from build123d import *

# Parameters (mm, degrees)
SWEEP1_PROFILE_R     = 13.49375
CUT_SWEEP1_PROFILE_R = 9.525


with BuildPart() as part:
    # Sweep1: sweep along a curve in space
    with BuildLine() as sweep1_path:
        Line((27.501516454, -11.100021656, -13.942942833), (23.095618699, 7.173839424, -10.851573197))
        add(Edge.make_bspline(
            [(23.095618699, 7.173839424, -10.851573197), (13.261070206, 47.963522462, -3.951225916), (-24.99522441, 69.205871428, 24.49264735), (-71.502710672, 110.316771936, -5.131837889)],
            knots=[0, 0, 0, 0, 1, 1, 1, 1], degree=3))
        Line((-71.502710672, 110.316771936, -5.131837889), (-88.677665299, 125.498797619, -16.07199464))
    # Sweep1 profile (on start of the path) → Sweep1 (sweep)
    with BuildSketch(Plane(origin=(27.501516454, -11.100021656, -13.942942833), x_dir=(0.9721432612515079, 0.2343874561560038, 0), z_dir=(-0.23128072205980535, 0.9592577994369071, 0.1622766213074379))):
        Circle(SWEEP1_PROFILE_R)
    sweep(path=sweep1_path.line)

    # Cut-Sweep1: sweep along a curve in space
    with BuildLine() as cut_sweep1_path:
        Line((27.501516454, -11.100021656, -13.942942833), (23.095618699, 7.173839424, -10.851573197))
        add(Edge.make_bspline(
            [(23.095618699, 7.173839424, -10.851573197), (13.261070206, 47.963522462, -3.951225916), (-24.99522441, 69.205871428, 24.49264735), (-71.502710672, 110.316771936, -5.131837889)],
            knots=[0, 0, 0, 0, 1, 1, 1, 1], degree=3))
        Line((-71.502710672, 110.316771936, -5.131837889), (-88.677665299, 125.498797619, -16.07199464))
    # Cut-Sweep1 profile (on start of the path) → Cut-Sweep1 (sweep, cut)
    with BuildSketch(Plane(origin=(27.501516454, -11.100021656, -13.942942833), x_dir=(0.9721432612515079, 0.2343874561560038, 0), z_dir=(-0.23128072205980535, 0.9592577994369071, 0.1622766213074379))):
        Circle(CUT_SWEEP1_PROFILE_R)
    sweep(path=cut_sweep1_path.line, mode=Mode.SUBTRACT)


solid = part.part
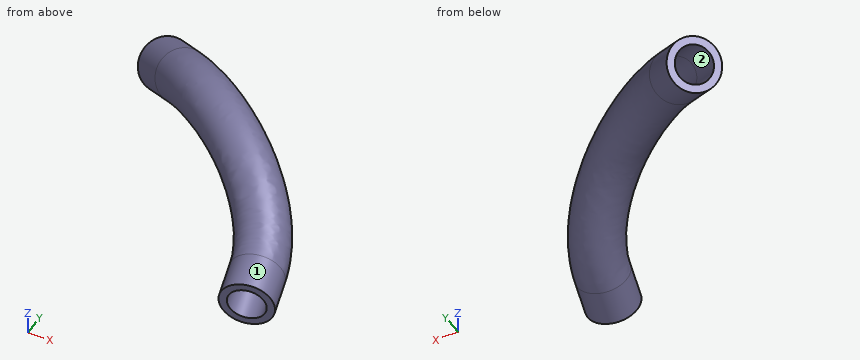
The model under review builds one solid part; all positions refer to its coordinate system, in mm. Face numbers are marked on the shaded views. Round coordinates to 2 decimals unless told otherwise and drop trailing zeros. Answer as CSV lines item,"result". Start each with the question number.
Q1. Clearance check with flat-ended pins moving along their axes: P1, Ø3, axis at y = 97, z = -11, coming from the -X side; P2, Ø8, axis at x = -11.5, z = -3, coming from the +Y side; P3, Ø6, axis at y = 19.5, z = -5, coming from the +X side. State where each tip first meets the part, or that it passes through.
Q2. Consider section A-A, the plane z = -6.5. State how many separate pieces and enclosed holes the cut face has, then the cut area to 3 significant figures.
Q3. Wall thickness on line 1 along Y through (x, z) = (-19, 2.5); line 2 along Y through (x, z) = (-9.5, 13.5); line 3 along X through (y, z) = (109.5, 1): over which ranges is each line inside the solid? List them lowest first.
Q4. The part is to be moulded in two halves that separate along Y. For the marked faces 1 and 2, say which applies: +Y half, -Y half, draft (parallel to the pull), parting line (faces both ways), or undercut.
Result set:
1,P1,"stops at x = -75.57"
1,P2,"stops at y = 76.8"
1,P3,"stops at x = 34"
2,separate pieces,"2"
2,enclosed holes,"1"
2,area,"1,630 mm²"
3,line 1,"y = 48.61 to 54.62, 76.64 to 82.46"
3,line 2,"y = 44.75 to 52.2, 66.65 to 73.86"
3,line 3,"x = -84.87 to -79, -56.08 to -49.91"
4,face 1,"parting line"
4,face 2,"undercut"
